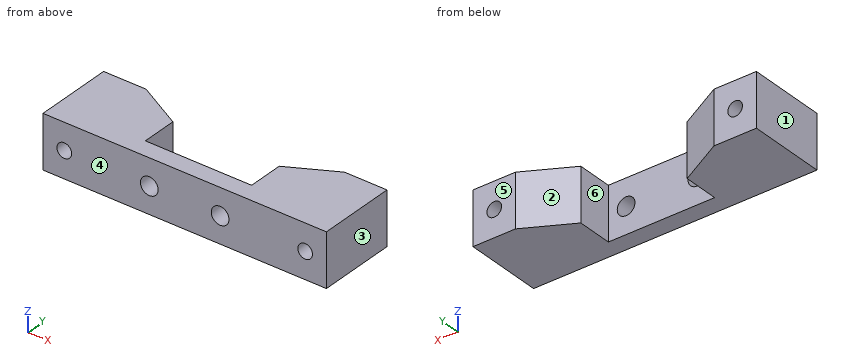
Autodesk Inventor part; units mm, degrees
ref_plane "YZ Plane" through (0, 0, 0) normal (1, 0, 0) x (0, 1, 0)
ref_plane "XZ Plane" through (0, 0, 0) normal (0, 1, 0) x (-1, 0, 0)
ref_plane "XY Plane" through (0, 0, 0) normal (0, 0, 1) x (1, 0, 0)
sketch "Sketch1" plane through (0, 0, 0) normal (0, 0, 1) x (1, 0, 0)
  line L0 (-36.9645, 19.732) -> (-36.9645, -2.268)
  line L1 (-36.9645, -2.268) -> (43.0355, -2.268)
  line L2 (43.0355, -2.268) -> (43.0355, 19.732)
  line L3 (43.0355, 19.732) -> (31.0355, 19.732)
  line L4 (31.0355, 19.732) -> (18.0355, 12.732)
  line L5 (18.0355, 12.732) -> (18.0355, 2.732)
  line L6 (18.0355, 2.732) -> (-11.9645, 2.732)
  line L7 (-11.9645, 2.732) -> (-11.9645, 12.732)
  line L8 (-11.9645, 12.732) -> (-24.9645, 19.732)
  line L9 (-24.9645, 19.732) -> (-36.9645, 19.732)
  dimension "d0" = 22
  dimension "d1" = 80
  dimension "d2" = 90
  dimension "d3" = 12
  dimension "d4" = 90
  dimension "d5" = 12
  dimension "d6" = 25
  dimension "d7" = 55
  dimension "d8" = 22
  dimension "d9" = 15
  dimension "d10" = 15
  dimension "d11" = 5
extrude "Extrusion1" add sketch "Sketch1" along normal blind 15
sketch "Sketch2" plane through (-36.9645, -2.268, 0) normal (0, -1, 0) x (1, 0, 0)
  line L0 (80, 15) -> (0, 15)
  line L1 (0, 0) -> (0, 15)
  circle A0 centre (30, 7.5) radius 2.5
  circle A1 centre (50, 7.5) radius 2.5
  point P0 (36.9645, 0)
  dimension "d14" = 5
  dimension "d17" = 20
  dimension "d22" = 30
  dimension "d23" = 7.5
extrude "Extrusion2" cut sketch "Sketch2" against normal through all
sketch "Sketch3" plane through (-36.9645, 19.732, 0) normal (0, 1, 0) x (1, 0, 0)
  line L0 (12, 0) -> (0, 0)
  line L1 (0, 0) -> (0, -15)
  line L2 (68, -15) -> (80, -15)
  line L3 (80, 0) -> (80, -15)
  line L4 (80, 0) -> (68, 0)
  line L5 (68, 0) -> (68, -15)
  circle A0 centre (6, -7.5) radius 2.5
  circle A1 centre (74, -7.5) radius 2.5
  point P0 (36.9645, 0)
  dimension "d26" = 5
  dimension "d27" = 7.5
  dimension "d28" = 6
  dimension "d29" = 5
  dimension "d30" = 6
  dimension "d31" = 7.5
hole "Hole1" at (-30.9645, 19.732, 7.5) at (37.0355, 19.732, 7.5) direction (0, -1, 0) diameter 4.134 end through all
equation "\"d8\" = d0"
equation "\"d31\" = d27"
properties part number "SM-TM1" material "Aluminum-6061"
Could you check a few things on this model? Use its own coordinates, in mm. Face numbers are marked on the shaded views. A direction names the side the tool comes from. Coordinates: 2 decimals unless noted, no trailing zeros. Order: outer loops, then holes, each group sorted by start corner. A loop starts at its lowest first (then second) coordinate and runs counter-clockwise, first axis right, second up. Notation, with made-up numbers: M -31.75,22.5 L 11.25,22.5 A25 ccw 11.25,46.5 Z; hole C -8,-16 d11. An arc over 180 degrees is marked long. Use one line per item in the form item = value. Start each with the question number.
1. Suppose I cut it at C-C on z = 11.5. Write out the boundary of the cut face in (x, y), then the cut area to 3 significant figures.
2. We'd pull the mould along X, two halves only. Please class the marked faces 1, 2, 3 and 4: +X half, -X half, draft (parallel to the pull), parting line (faces both ways), or undercut.
3. For pin 1 (3 mm diameter, centred on x = -5.5, y = 4, fed in from +Z); pin 2 (3.5 mm diameter, centred on x = 37.04, z = 7.5, fed in from +Y); pin 3 (8 mm diameter, centred on x = -6.96, z = 7.5, fed in from +Y), each with a flat end and sliding along its axis, tell me the tip position at first contact or that it passes through.
4. On a 3-axis mill with a long thin cutter (end or side, diameter ignored), from which of +Z, -Z, +X, -X, +Y, -Y can I reach the whole of each face in a straight line? I mean the marked faces 5 and 6. Say none if no direction works.
5. Please list where these lines run through material, in increasing order: line 1 (X direction, y = 11, z = 7.5); line 2 (X direction, y = 0.75, z = 6); line 3 (X direction, y = 15.5, z = 7.5).
6. Suppose I cut it at B-B on y = 15.25. Write out the boundary of the cut face in (x, z), then the cut area to 3 significant figures.
7. Suppose I cut it at A-A on z = 7.5. Write out the boundary of the cut face in (x, y), then the cut area to 3 significant figures.
8. Suppose I cut it at D-D on y = 1. Write out the boundary of the cut face in (x, z).
Geometry says:
q1.outline = M -36.96,-2.27 L 43.04,-2.27 L 43.04,19.73 L 31.04,19.73 L 18.04,12.73 L 18.04,2.73 L -11.96,2.73 L -11.96,12.73 L -24.96,19.73 L -36.96,19.73 Z
q1.area = 1,160 mm^2
q2.face_1 = -X half
q2.face_2 = undercut
q2.face_3 = +X half
q2.face_4 = draft
q3.pin_1 = 15
q3.pin_2 = through
q3.pin_3 = 2.73
q4.face_5 = +Z, -Z, +X, -X, +Y
q4.face_6 = +Z, -Z, +Y
q5.line_1 = -36.96 to -33.03, -28.9 to -11.96, 18.04 to 34.97, 39.1 to 43.04
q5.line_2 = -36.96 to -32.39, -29.54 to -8.96, -4.96 to 11.04, 15.04 to 35.61, 38.46 to 43.04
q5.line_3 = -36.96 to -33.03, -28.9 to -17.11, 23.18 to 34.97, 39.1 to 43.04
q6.outline = M -36.96,0 L -16.64,0 L -16.64,15 L -36.96,15 Z; M 22.71,0 L 43.04,0 L 43.04,15 L 22.71,15 Z; hole C -30.96,7.5 d4.13; hole C 37.04,7.5 d4.13
q6.area = 583 mm^2
q7.outline = M -36.96,-2.27 L -33.03,-2.27 L -33.03,19.73 L -36.96,19.73 Z; M -28.9,-2.27 L -9.46,-2.27 L -9.46,2.73 L -11.96,2.73 L -11.96,12.73 L -24.96,19.73 L -28.9,19.73 Z; M -4.46,-2.27 L 10.54,-2.27 L 10.54,2.73 L -4.46,2.73 Z; M 15.54,-2.27 L 34.97,-2.27 L 34.97,19.73 L 31.04,19.73 L 18.04,12.73 L 18.04,2.73 L 15.54,2.73 Z; M 39.1,-2.27 L 43.04,-2.27 L 43.04,19.73 L 39.1,19.73 Z
q7.area = 927 mm^2
q8.outline = M -36.96,0 L 43.04,0 L 43.04,15 L -36.96,15 Z; hole C -30.96,7.5 d4.13; hole C -6.96,7.5 d5; hole C 13.04,7.5 d5; hole C 37.04,7.5 d4.13
